Verification items for the finished model (mm, model axes). Face numbers are marked on the shaded views. A direction names the side the tool comes from. Give positions to 0.01 mm unless a question says otherwise; leave off trailing zeros. Order: outer loops, then holes, each group sorted by start corner. A loop starts at its lowest first (then second) coordinate and runs counter-clockwise, first axis right, second up.
(1) Sectioned sample at A-A on z = 24. Record the cut outline in (x, y), plus the area to 3 significant figures.
(2) Gauge pin test, flat ends, axial feed: pin 1 (3 mm diameter, centred on x = 10, z = 6.5, fed in from +Y); pin 2 (3 mm diameter, centred on x = 1, y = -20, fed in from +Z); pin 3 (2.5 mm diameter, centred on y = 0, z = -3.81, fed in from +X). Record the tip position at first contact, or that the pin passes through.
(3) Mould release check, pull along X, two halves, no side actions. Record for the marked faces 1, 2 and 3: pulls with the +X half, pulls with the -X half, needs draft (parallel to the pull), parting line crosses it, or undercut.
(4) Access from +Z, -Z, +X, -X, +Y, -Y to the whole of each face (thin tool, end or side, straight path). Record for the marked faces 4, 5 and 6.
(5) Scan lines: L1, parallel to Z at x = -4.55, y = 0; L2, parallel to Y at x = 0, z = -3.75 (1 decimal); L3, parallel to Y at x = 0, z = -9 (3 decimals). Record each from-to range of solid material in increasing order.
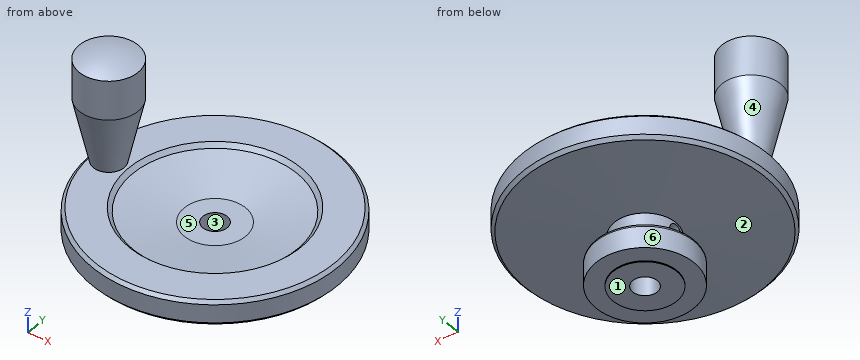
```python
from build123d import *
from OCP.BRepFilletAPI import BRepFilletAPI_MakeChamfer

# Parameters (mm, degrees)
SKETCH1_R                   = 31.75
EXTRUDE1_DEPTH              = 6.35
SKETCH4_R                   = 7.9375
EXTRUDE2_DEPTH              = 6.35
SKETCH5_R                   = 12.7
EXTRUDE3_DEPTH              = 6.35
SKETCH6_R                   = 8.255
EXTRUDE4_DEPTH              = 0.254
SKETCH7_R                   = 3.175
EXTRUDE5_DEPTH              = 50.390428992
FILLET1_R                   = 0.79375
CHAMFER1_SIZE               = 0.79375
CHAMFER1_SIZE2              = 0.839659951
F_10_32_TAPPED_HOLE1_REACH  = 53.959
F_10_32_TAPPED_HOLE1_BORE_R = 2.0193
SKETCH12_R                  = 3.175
EXTRUDE6_DEPTH              = 27.94


with BuildPart() as part:
    # Sketch1 → Extrude1 (new body)
    with BuildSketch(Plane.XY):
        Circle(SKETCH1_R)
    extrude(amount=EXTRUDE1_DEPTH)

    # Sketch2 → Cut-Revolve4 (revolve, cut)
    with BuildSketch(Plane(origin=(0, 0, 0), x_dir=(1, 0, 0), z_dir=(0, 1, 0)), mode=Mode.PRIVATE) as cut_revolve4_sk:
        Polygon((22.225, -6.35), (21.209, -5.334), (7.9375, -2.54), (0, -2.54), (0, -6.35), align=None)
    revolve(cut_revolve4_sk.sketch.rotate(Axis((0, 0, 0), (0, 0, 1)), 180), axis=Axis((0, 0, 0), (0, 0, 1)), mode=Mode.SUBTRACT)

    # Sketch3 → Revolve1 (revolve)
    with BuildSketch(Plane(origin=(0, 0, 0), x_dir=(1, 0, 0), z_dir=(0, 1, 0)), mode=Mode.PRIVATE) as revolve1_sk:
        Polygon((-31.75, 0), (-7.9375, 1.27), (0, 1.27), (0, 0), align=None)
    revolve(revolve1_sk.sketch.rotate(Axis((0, 0, 0), (0, 0, -1)), 180), axis=Axis((0, 0, 0), (0, 0, -1)))

    # Sketch4 → Extrude2 (add)
    with BuildSketch(Plane(origin=(0, 0, -1.27), x_dir=(-1, 0, 0), z_dir=(0, 0, -1))):
        with Locations(Location((0, 0, 0), (0, 0, 180))):
            Circle(SKETCH4_R)
    extrude(amount=EXTRUDE2_DEPTH)

    # Sketch5 → Extrude3 (add)
    with BuildSketch(Plane(origin=(0, 0, -7.62), x_dir=(-1, 0, 0), z_dir=(0, 0, -1))):
        with Locations(Location((0, 0, 0), (0, 0, 180))):
            Circle(SKETCH5_R)
    extrude(amount=EXTRUDE3_DEPTH)

    # Sketch6 → Extrude4 (add)
    with BuildSketch(Plane(origin=(0, 0, -13.97), x_dir=(-1, 0, 0), z_dir=(0, 0, -1))):
        with Locations(Location((0, 0, 0), (0, 0, 180))):
            Circle(SKETCH6_R)
    extrude(amount=EXTRUDE4_DEPTH)

    # Sketch7 → Extrude5 (cut, through all)
    with BuildSketch(Plane(origin=(0, 0, -14.224), x_dir=(-1, 0, 0), z_dir=(0, 0, -1))):
        Circle(SKETCH7_R)
    extrude(amount=-EXTRUDE5_DEPTH, mode=Mode.SUBTRACT)

    # Fillet1
    fillet1_edges = [part.edges().sort_by_distance(p)[0] for p in [
        (-12.7, 0, -7.62),
    ]]
    fillet(fillet1_edges, radius=FILLET1_R)

    # Chamfer1: one chamfer whose edges measure the first distance from different faces: ONE call of the kernel's chamfer builder (chamfer() names one face for all edges)
    chamfer1_edges_1 = [part.edges().sort_by_distance(p)[0] for p in [
        (-31.75, 0, 6.35),
    ]]
    chamfer1_edges_2 = [part.edges().sort_by_distance(p)[0] for p in [
        (-31.75, 0, 0),
    ]]
    chamfer1_side_2 = [part.faces().sort_by_distance(p)[0] for p in [
        (-19.84375, 0, -0.635),
    ]]
    chamfer1 = BRepFilletAPI_MakeChamfer(part.part.solid().wrapped)
    for e in chamfer1_edges_1:
        chamfer1.Add(CHAMFER1_SIZE, e.wrapped)
    for e in chamfer1_edges_2:
        chamfer1.Add(CHAMFER1_SIZE, CHAMFER1_SIZE2, e.wrapped, chamfer1_side_2[0].wrapped)  # the first distance lies on this face
    add(Compound.cast(chamfer1.Shape()), mode=Mode.REPLACE)

    # #10-32 Tapped Hole1 bore → #10-32 Tapped Hole1 (cut, up to next)
    with BuildSketch(Plane(origin=(-7.9375, 0, -4.445), x_dir=(0, -1, 0), z_dir=(-1, 0, 0)), mode=Mode.PRIVATE) as f_10_32_tapped_hole1_sk1:
        with Locations((0, 0.635)):
            Circle(F_10_32_TAPPED_HOLE1_BORE_R)
    f_10_32_tapped_hole1_tool1 = extrude(f_10_32_tapped_hole1_sk1.sketch, amount=-F_10_32_TAPPED_HOLE1_REACH, mode=Mode.PRIVATE) & part.part
    add(f_10_32_tapped_hole1_tool1.solids().sort_by_distance((-7.9375, 0, -3.81))[0], mode=Mode.SUBTRACT)

    # Sketch12 → Extrude6 (add)
    with BuildSketch(Plane.XY.offset(6.35)):
        with Locations((-26.9875, 0)):
            Circle(SKETCH12_R)
    extrude(amount=EXTRUDE6_DEPTH)

    # Sketch13 → Revolve2 (revolve)
    with BuildSketch(Plane(origin=(0, 0, 0), x_dir=(1, 0, 0), z_dir=(0, 1, 0)), mode=Mode.PRIVATE) as revolve2_sk:
        with BuildLine():
            Line((-26.9875, -6.35), (-23.01875, -6.35))
            Line((-23.01875, -6.35), (-19.3675, -22.808497077))
            Line((-19.3675, -22.808497077), (-19.3675, -32.968497077))
            ThreePointArc((-19.3675, -32.968497077), (-23.095695912, -34.154906701), (-26.9875, -34.555997077))
            Line((-26.9875, -34.555997077), (-26.9875, -6.35))
        make_face()
    revolve(revolve2_sk.sketch.rotate(Axis((-26.9875, 0, -6.630939357), (0, 0, 1)), 180), axis=Axis((-26.9875, 0, -6.630939357), (0, 0, 1)))


solid = part.part
```
Ans:
1. outline: circle Ø15.24 at (-26.99, 0)
1. area: 182 mm2
2. pin 1: stops at y = 30.5
2. pin 2: stops at z = 5.65
2. pin 3: stops at x = 7.94
3. face 1: needs draft
3. face 2: parting line crosses it
3. face 3: undercut
4. face 4: none
4. face 5: +Z
4. face 6: -Z
5. L1: z = -14.22 to -5.83, -1.79 to 2.54
5. L2: y = -7.9 to -3.2, 3.2 to 7.9
5. L3: y = -12.7 to -3.175, 3.175 to 12.7
